Input: part model. Units: mm. Frame: model coordinates. A direction names the side the tool comes from. Coordinates: 2 decimals unless noted, no trailing zeros. Write each loop counter-clockwise with the first axis right and the second up, starting at its lowest first coordinate (ties: lowest second). Pieces come first, ordered by that corner, then holes.
1) Draft query along X for faces 3 (the flat face through (330.2, 122, 14)), 4 (the flat face through (-311.15, 132, 14)), 5 (the flat face through (-314, 97, 1022.35)). Return one class per face: pulls with the +X half, pulls with the -X half, needs draft (parallel to the pull), parting line crosses it, or undercut.
2) Line query: L1, parallel to X at y = 45, z = -844; L2, parallel to Y at x = -39.5, z = 163. Output: solid intervals per line, ascending.
3) Pin query (flat end, axial travel): pin 1 Ø3 at (x, z) = (147.5, -290.5) entering from +Y; pin 2 Ø15 at (x, y) = (34, 8.5) entering from +Z; pin 3 Ø15 at (x, y) = (166, 12.5) entering from +Z. Return the tip coordinate at first contact, or that it passes through.
4) Section query D-D (x = -77). Output: boundary loops of the cut face in (y, z).
5) Section query C-C (z = 201.5). Output: boundary loops of the cut face in (x, y), then the cut area to 3 significant figures.
6) Section query A-A (z = 882.5). Output: boundary loops of the cut face in (x, y), then the cut area to 3 significant figures.
7) Set-up query: faces 1 (the flat face through (313, 88, 1022.35)), 2 (the flat face through (311.15, 135, 14)). Return all of +Z, -Z, +X, -X, +Y, -Y with unobstructed straight access to the full face (end or side cutting, diameter ignored); none if empty.
8) Section query B-B (y = 56.5). Output: boundary loops of the cut face in (x, z).
from build123d import *

# Parameters (mm, degrees)
F1_DEPTH = 1022.35
F3_DEPTH = 25.4


with BuildPart() as f1:
    # F0 (on Top) → F1 (new body, symmetric)
    with BuildSketch(Plane.XY):
        Polygon((311.15, 247.65), (311.15, 19.05), (-311.15, 19.05), (-311.15, 247.65), (-330.2, 247.65), (-330.2, 0), (330.2, 0), (330.2, 247.65), align=None)
    extrude(amount=F1_DEPTH, both=True)

    # F2 (on face) → F3 (cut)
    with BuildSketch(Plane.XZ):
        Polygon((203.2, 1022.35), (-203.2, 1022.35), (-203.2, 768.35), (-152.4, 768.35), (-152.4, 666.75), (152.4, 666.75), (152.4, 768.35), (203.2, 768.35), align=None)
    extrude(amount=-F3_DEPTH, mode=Mode.SUBTRACT)


solid = f1.part
Answer:
1. face 3: pulls with the +X half
1. face 4: undercut
1. face 5: needs draft
2. L1: x = -330.2 to -311.15, 311.15 to 330.2
2. L2: y = 0 to 19.05
3. pin 1: stops at y = 19.05
3. pin 2: stops at z = 666.75
3. pin 3: stops at z = 768.35
4. outline: (0, -1022.35) - (19.05, -1022.35) - (19.05, 666.75) - (0, 666.75) - close
5. outline: (-330.2, 0) - (330.2, 0) - (330.2, 247.65) - (311.15, 247.65) - (311.15, 19.05) - (-311.15, 19.05) - (-311.15, 247.65) - (-330.2, 247.65) - close
5. area: 21,300 mm2
6. outline: (-330.2, 0) - (-203.2, 0) - (-203.2, 19.05) - (-311.15, 19.05) - (-311.15, 247.65) - (-330.2, 247.65) - close; (203.2, 0) - (330.2, 0) - (330.2, 247.65) - (311.15, 247.65) - (311.15, 19.05) - (203.2, 19.05) - close
6. area: 13,500 mm2
7. face 1: +Z, +X, -X, +Y, -Y
7. face 2: +Z, -Z, +Y
8. outline: (-330.2, -1022.35) - (-311.15, -1022.35) - (-311.15, 1022.35) - (-330.2, 1022.35) - close; (311.15, -1022.35) - (330.2, -1022.35) - (330.2, 1022.35) - (311.15, 1022.35) - close
